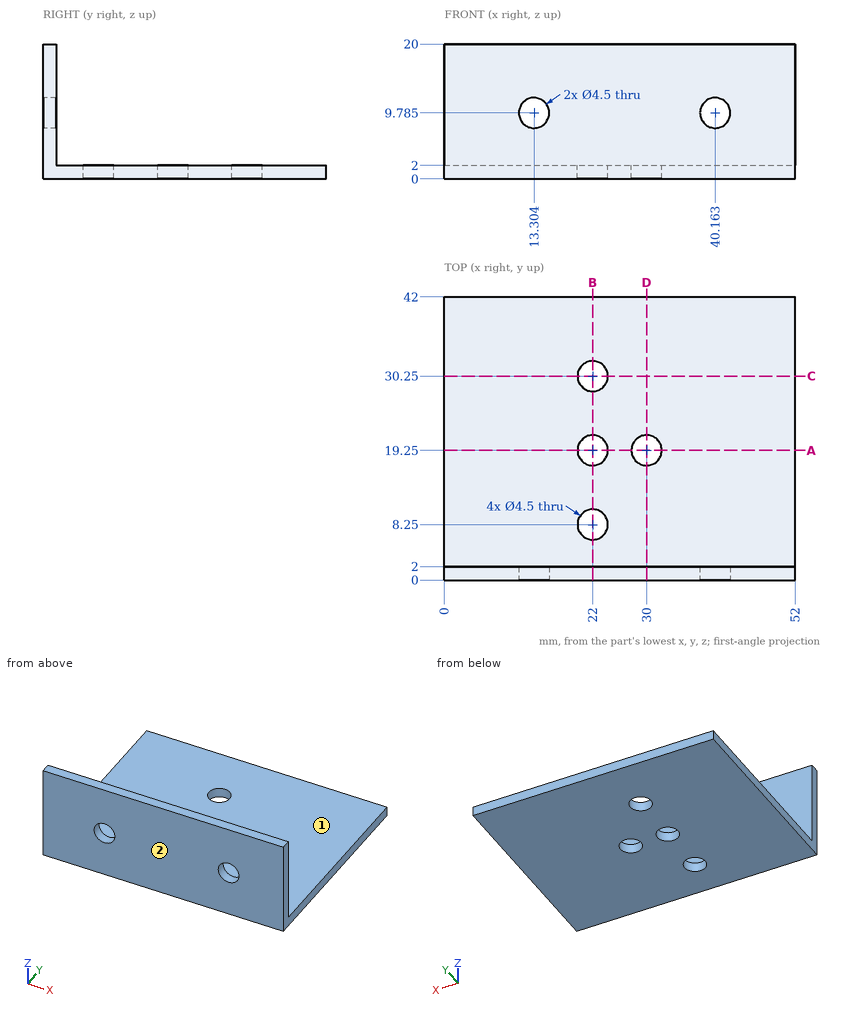
Design review of the part shown in the three views and the two pictorial views. Dimensions are in mm from the part's minimum x, y and z. A direction names the side the tool comes from. Give positions to 0.01 mm unless a question says otherwise; leave off trailing zeros. Write each loop counter-clockwise with the first axis right and the second up, starting at its lowest first coordinate (ties: lowest second). Pieces come first, ordered by that corner, then holes.
Item 1: Machinability: for the marked faces 1 and 2, which of the approach directions +Z, -Z, +X, -X, +Y, -Y give a long, thin tool a straight path to every point of the face, cutting with its end or side? Answer none if there is none.
Item 2: Take a section at D-D (x = 30). Give the boundary of the cut face in (y, z), and give its area (3 significant figures).
Item 3: Take a section at B-B (x = 22). Give the boundary of the cut face in (y, z).
Item 4: Take a section at A-A (y = 19.25). Give the boundary of the cut face in (x, z).
Item 5: Insertion check: P1, Ø2, axis at x = 42.5, y = 34.5, coming from the +Z side; P2, Ø5.5, axis at x = 33.5, z = 10, coming from the +Y side. Each pin has a flat end and moves straight along its axis. Give the tip position at first contact, or say it passes through.
Item 6: Take a section at C-C (y = 30.25). Give the boundary of the cut face in (x, z).
Item 7: Wall thickness on probe 1 along Y at (x, z) = (22, 1.1); probe 2 along Y at (x, z) = (30, 0.8); probe 3 along Z at (x, y) = (36, 12): over which ranges is each line inside the solid? List them lowest first.
Established:
1. face 1: +Z, +X, -X, +Y
1. face 2: +Z, -Z, +X, -X, -Y
2. outline: (0, 0) - (17, 0) - (17, 2) - (2, 2) - (2, 20) - (0, 20) - close; (21.5, 0) - (42, 0) - (42, 2) - (21.5, 2) - close
2. area: 111 mm2
3. outline: (0, 0) - (6, 0) - (6, 2) - (2, 2) - (2, 20) - (0, 20) - close; (10.5, 0) - (17, 0) - (17, 2) - (10.5, 2) - close; (21.5, 0) - (28, 0) - (28, 2) - (21.5, 2) - close; (32.5, 0) - (42, 0) - (42, 2) - (32.5, 2) - close
4. outline: (0, 0) - (19.75, 0) - (19.75, 2) - (0, 2) - close; (24.25, 0) - (27.75, 0) - (27.75, 2) - (24.25, 2) - close; (32.25, 0) - (52, 0) - (52, 2) - (32.25, 2) - close
5. P1: stops at z = 2
5. P2: stops at y = 2
6. outline: (0, 0) - (19.75, 0) - (19.75, 2) - (0, 2) - close; (24.25, 0) - (52, 0) - (52, 2) - (24.25, 2) - close
7. probe 1: y = 0 to 6, 10.5 to 17, 21.5 to 28, 32.5 to 42
7. probe 2: y = 0 to 17, 21.5 to 42
7. probe 3: z = 0 to 2
